Can you work these out from the model? Positions are in its coordinate system, mm. Give positions to 0.01 mm unless a question says otherwise; leave off trailing zeros. Answer as a JSON object with one key per item and string values.
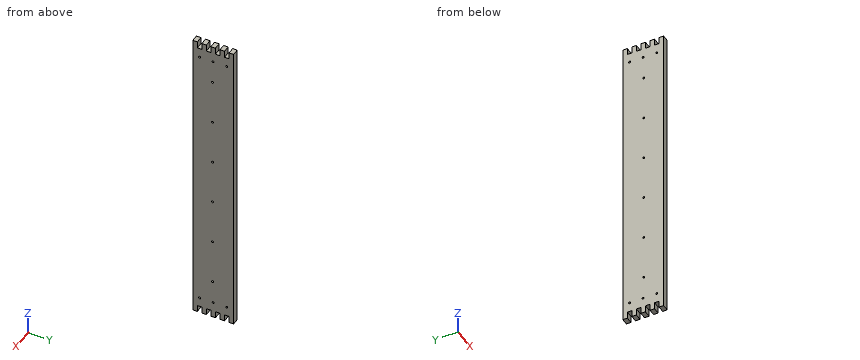
```python
from build123d import *

# Parameters (mm, degrees)
BOSS_EXTRUDE1_DEPTH             = 19.05
F_7_32_0_21875_DIAMETER_HOLE2_D = 5.55625


with BuildPart() as part:
    # Sketch1 → Boss-Extrude1 (new body)
    with BuildSketch(Plane(origin=(0, 0, 0), x_dir=(0, 0, -1), z_dir=(1, 0, 0))):
        Polygon((0, 0), (862.33, 0), (862.33, 12.7), (843.28, 12.7), (843.28, 25.4), (862.33, 25.4), (862.33, 38.1), (843.28, 38.1), (843.28, 50.8), (862.33, 50.8), (862.33, 63.5), (843.28, 63.5), (843.28, 76.2), (862.33, 76.2), (862.33, 88.9), (843.28, 88.9), (843.28, 101.6), (862.33, 101.6), (862.33, 114.3), (0, 114.3), (0, 101.6), (19.05, 101.6), (19.05, 88.9), (0, 88.9), (0, 76.2), (19.05, 76.2), (19.05, 63.5), (0, 63.5), (0, 50.8), (19.05, 50.8), (19.05, 38.1), (0, 38.1), (0, 25.4), (19.05, 25.4), (19.05, 12.7), (0, 12.7), align=None)
    extrude(amount=BOSS_EXTRUDE1_DEPTH)

    # 7/32 (0.21875) Diameter Hole2 (through all)
    with Locations(Plane(origin=(19.05, 0, 0), x_dir=(0, 0, -1), z_dir=(1, 0, 0))):
        with Locations((816.4449, 57.15), (112.5601, 55.499), (240.00206, 55.499), (367.44402, 55.499), (494.88598, 55.499), (622.32794, 55.499), (749.7699, 55.499), (816.4449, 95.25), (816.4449, 19.05), (45.8851, 95.25), (45.8851, 19.05), (45.8851, 57.15)):
            Hole(F_7_32_0_21875_DIAMETER_HOLE2_D / 2)


solid = part.part
```
1. Will these pins go through, and if not, where does the flat tip stop? pin 1 Ø6.5 at (x, y) = (13.5, 46) entering from -Z; pin 2 Ø4 at (x, y) = (7, 19) entering from +Z.
Worked answers:
{"pin 1": "z = -843.28", "pin 2": "z = -19.05"}
2. If we section it at A-A on x = 5.75: Count the separate pieces of the cut face and the enclosed holes in it, then the cut area to 3 significant figures.
Worked answers:
{"separate pieces": "1", "enclosed holes": "12", "area": "96,300 mm²"}
3. Please list where these lines run through material, in increasing order: L1, parallel to Y at x = 14.5, z = -114; L2, parallel to Z at x = 1.75, y = 66.
Worked answers:
{"L1": "0 to 53.12, 57.87 to 114.3", "L2": "-843.28 to -19.05"}
